Source: CAD feature listing. Evaluate the final solid. Frame: model axes, mm. A direction names the side the tool comes from. Round coordinates to 2 decimals unless told otherwise and drop trailing zeros. Loops run counter-clockwise (first coordinate to the right, second up) from the corner with the lowest first, then second, coordinate; pieces in that order, holes last. Notation, with made-up numbers: (44, -4.5) - (60, -4.5) arc R16 cw to (60, 18.5) - close; hole circle Ø9 at (44, 47.5). An arc over 180 degrees is marked (long way). Write item = value, one per line. Start each with the question number.
Autodesk Inventor part; units mm, degrees
ref_plane "YZ Plane" through (0, 0, 0) normal (1, 0, 0) x (0, 1, 0)
ref_plane "XZ Plane" through (0, 0, 0) normal (0, 1, 0) x (-1, 0, 0)
ref_plane "XY Plane" through (0, 0, 0) normal (0, 0, 1) x (1, 0, 0)
sketch "Sketch1" plane through (0, 0, 0) normal (0, 0, 1) x (1, 0, 0)
  line L0 (-28.59, -15) -> (28.59, -15)
  line L1 (28.59, -15) -> (28.59, 15)
  line L2 (28.59, 15) -> (-28.59, 15)
  line L3 (-28.59, 15) -> (-28.59, -15)
  line L4 (-28.59, -15) -> (28.59, 15) construction
  line L5 (28.59, -15) -> (-28.59, 15) construction
  point P0 (0, 0)
  dimension "d0" = 57.18
  dimension "d1" = 30
extrude "Plate1" add sketch "Sketch1" along normal blind 1.5
sketch "Sketch2" plane through (-27.09, -15, 0) normal (-1, 0, 0) x (0, -1, 0)
  line L0 (-30, 0) -> (0, 0)
  line L1 (0, 0) -> (0, 45)
  line L2 (0, 45) -> (-30, 45)
  line L3 (-30, 45) -> (-30, 0)
edge flange "Flange1" height 45 angle 90 thickness 1.5 bend radius 0.31 thickness toward (-1, 0, 0) relief tear relief width 1.5 relief depth 0.75 corner gap 0.31 corner form 0 edges at (-28.59, 0, 1.5) (28.59, 0, 1.5) wall of the first edge with corners at (-27.09, 15, 0) (-27.09, -15, 0) (-27.09, -15, 45) (-27.09, 15, 45)
bend "Bend1"
corner "Corner1"
sketch "Sketch3" plane through (28.59, -15, 45) normal (1, 0, 0) x (0, 0, -1)
  circle A0 centre (17, 15) radius 9.96
  line L0 (0, 30) -> (43.19, 30)
  line L1 (43.19, 0) -> (0, 0)
  line L2 (31.19, 30) -> (13.9636, 24.4859)
  line L3 (31.19, 0) -> (13.9636, 5.5141)
  line L4 (0, 30) -> (0, 0)
  point P0 (45, 15)
  dimension "d13" = 19.92
  dimension "d14" = 12
  dimension "d15" = 28
extrude "Cut1" cut sketch "Sketch3" against normal blind 57.18 contours A0 L3 L1 L4 L0 L2
sketch "Sketch4" plane through (0, 0, 1.5) normal (0, 0, 1) x (1, 0, 0)
  circle A0 centre (7, 0) radius 0.7835
  circle A1 centre (0, -7) radius 0.7835
  circle A2 centre (-7, 0) radius 0.7835
  circle A3 centre (0, 7) radius 0.7835
  circle A4 centre (0, 0) radius 2.925
hole "Hole1" at (7, 0, 1.5) at (0, 7, 1.5) at (-7, 0, 1.5) at (0, -7, 1.5) direction (0, 0, -1) diameter 2.1 depth 1.5
sketch "Sketch5" plane through (0, 0, 1.5) normal (0, 0, 1) x (1, 0, 0)
  circle A0 centre (0, 0) radius 1.75
  circle A1 centre (0, 0) radius 2.6
  point P0 (0, 0)
  dimension "d26" = 5.2
extrude "Extrusion1" cut sketch "Sketch5" against normal through all contours A0 | A1
sketch "Sketch12" plane through (28.59, -15, 1.81) normal (1, 0, 0) x (0, 0, -1)
  arc A0 (-29.2264, 24.4859) -> (-29.2264, 5.5141) centre (-26.19, 15) ccw
  circle A1 centre (-26.19, 15) radius 2.6
  circle A2 centre (-33.19, 15) radius 1.05
  circle A3 centre (-26.19, 8) radius 1.05
  circle A4 centre (-19.19, 15) radius 1.05
  circle A5 centre (-26.19, 22) radius 1.05
  point P0 (1.81, 15)
  dimension "d52" = 5.2
  dimension "d53" = 2.1
  dimension "d54" = 7
  dimension "d57" = 360
extrude "Cut5" cut sketch "Sketch12" against normal blind 57.18
sketch "Sketch13" plane through (28.59, -15, 1.81) normal (1, 0, 0) x (0, 0, -1)
  circle A0 centre (-26.19, 15) radius 2.6
  circle A1 centre (-26.19, 15) radius 3.6
  point P0 (1.81, 15)
  dimension "d61" = 7.2
extrude "Cut6" cut sketch "Sketch13" against normal blind 1.5
equation "\"d24\" = Thickness"
equation "\"d62\" = Thickness"
equation "\"d2\" = Thickness"
equation "\"d3\" = BendReliefWidth"
equation "\"d4\" = BendReliefDepth"
equation "\"d5\" = MinimumRemnant"
equation "\"d6\" = TransitionRadius"
equation "\"d9\" = BendRadius"
equation "\"d10\" = CornerReliefSize"
equation "\"d11\" = GapSize"
equation "\"d12\" = JacobiRadiusSize"
equation "\"BendReliefWidth\" = Thickness"
equation "\"BendReliefDepth\" = 0.5 * Thickness"
equation "\"CornerReliefSize\" = 4 * Thickness"
equation "\"MinimumRemnant\" = 2 * Thickness"
equation "\"TransitionRadius\" = BendRadius"
equation "\"JacobiRadiusSize\" = BendRadius"
equation "\"GapSize\" = Thickness"
properties part number "axis_5_bottom_frame" material "Aluminum 6061-AHC"
(1) Mould query, pull axis Y, two halves, no side actions, for faces 3 (the face through (27.85, 0.05, 36.05)), 4 (the face through (0, 4, 1.5)), 5 (the face through (0, 15, 1)). Classes: +Y half, -Y half, draft (parallel to the pull), parting line (faces both ways), or undercut.
(2) Pin query (flat end, axial travel): P1, Ø2, axis at x = -11.5, y = 9.5, coming from the +Z side; P2, Ø6.5, axis at y = 0, z = 28, coming from the +X side. Return the tip coordinate at first contact, or that it passes through.
(3) Material intervals for line 1 along Y through (x, z) = (-27.5, 28); line 2 along X through (y, z) = (8.5, 18.5); line 3 along Z through (x, y) = (-20.5, 11.5), sorted ascending. Write a range as from..to.
(4) Cut plane D-D (y = 7). Output: boundary loops of the cut face in (x, z).
(5) Cut plane C-C (z = 28). State how many separate pieces and enclosed holes the cut face has, and give its area (3 significant figures).
(6) Access query for faces 1 (the face through (27.09, 0, 16)), 2 (the face through (27.85, 12.282, 22.303)). Directions: +Z, -Z, +X, -X, +Y, -Y. A direction counts if a zero-diameter tool reaches every point of the face in a straight line with its end or side. Return the directions, or none.
(7) Cut plane B-B (x = 7). Output: boundary loops of the cut face in (y, z), and give its area (4 significant figures).
(8) Cut plane A-A (z = 8). Output: boundary loops of the cut face in (x, y).
Solution:
q1.face_3 = undercut
q1.face_4 = draft
q1.face_5 = +Y half
q2.P1 = 1.5
q2.P2 = -27.09
q3.line_1 = -10.46..-8.05, -5.95..-2.6, 2.6..5.95, 8.05..10.46
q3.line_2 = -28.59..-27.09, 27.09..28.59
q3.line_3 = 0..1.5
q4.outline = (-28.59, 1.81) arc R1.81 ccw to (-26.78, 0) - (-1.05, 0) - (-1.05, 1.5) - (-26.78, 1.5) arc R0.31 cw to (-27.09, 1.81) - (-27.09, 26.95) - (-28.59, 26.95) - close; (-28.59, 29.05) - (-27.09, 29.05) - (-27.09, 35.09) - (-28.59, 35.09) - close; (1.05, 0) - (26.78, 0) arc R1.81 ccw to (28.59, 1.81) - (28.59, 26.95) - (27.09, 26.95) - (27.09, 1.81) arc R0.31 cw to (26.78, 1.5) - (1.05, 1.5) - close; (27.09, 29.05) - (28.59, 29.05) - (28.59, 35.09) - (27.09, 35.09) - close
q5.separate_pieces = 8
q5.enclosed_holes = 0
q5.area = 31.5 mm^2
q6.face_1 = +Z, +Y, -Y
q6.face_2 = +Z, +X, -X, +Y
q7.outline = (-15, 0) - (-1.05, 0) - (-1.05, 1.5) - (-15, 1.5) - close; (1.05, 0) - (15, 0) - (15, 1.5) - (1.05, 1.5) - close
q7.area = 41.85 mm^2
q8.outline = (-28.59, -15) - (-27.09, -15) - (-27.09, 15) - (-28.59, 15) - close; (27.09, -15) - (28.59, -15) - (28.59, 15) - (27.09, 15) - close
